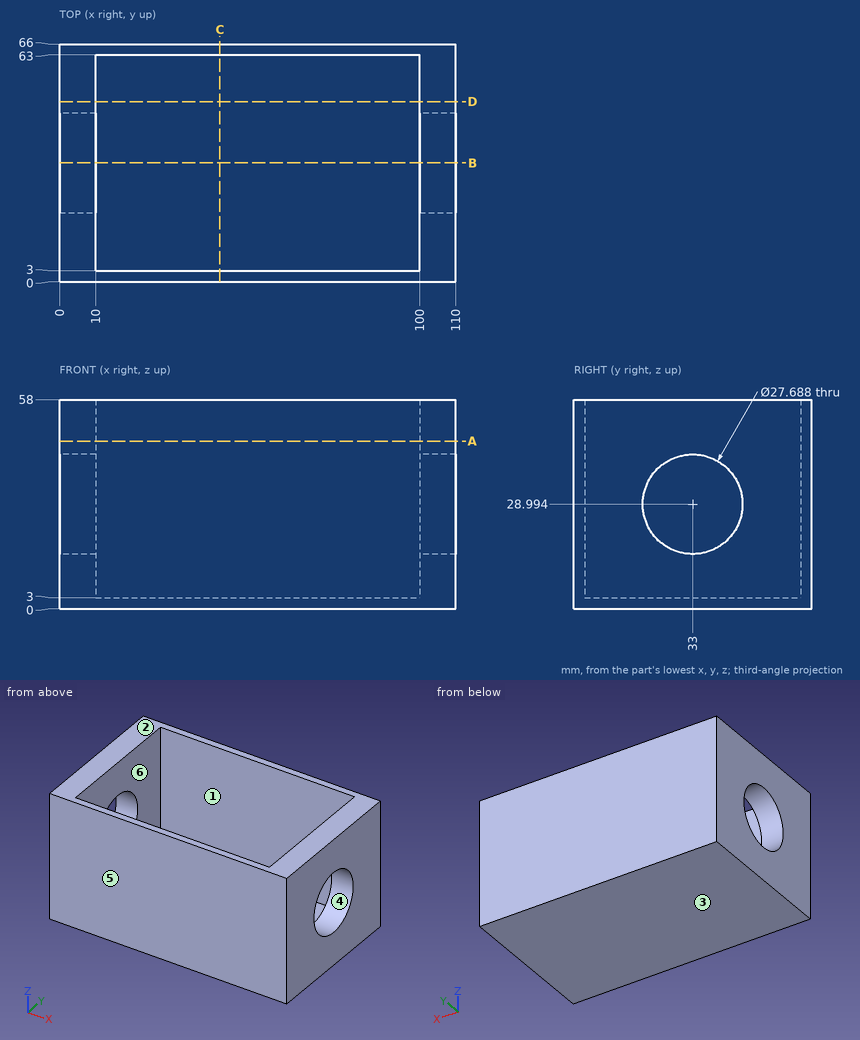
Here's the drawing with two shaded views (mm, measured from the low corner). I have some questions. A direction names the side the tool comes from. Round coordinates to 2 decimals unless told otherwise and drop trailing zeros. Loops run counter-clockwise (first coordinate to the right, second up) from the corner with the lowest first, then second, coordinate; pieces in that order, holes last. Notation, with made-up numbers: (-15, 34) - (37, 34) arc R25 cw to (37, 55) - close; hole circle Ø3 at (21, 1.25). An arc over 180 degrees is marked (long way). Write item = value, one per line.
1) Imagine slicing it at B-B (y = 33). Please give me the cut outline in (x, z).
Computed:
outline = (0, 0) - (110, 0) - (110, 15.15) - (100, 15.15) - (100, 3) - (10, 3) - (10, 15.15) - (0, 15.15) - close; (0, 42.84) - (10, 42.84) - (10, 58) - (0, 58) - close; (100, 42.84) - (110, 42.84) - (110, 58) - (100, 58) - close
2) Imagine slicing it at C-C (x = 44.5). Please give me the cut outline in (y, z).
Computed:
outline = (0, 0) - (66, 0) - (66, 58) - (63, 58) - (63, 3) - (3, 3) - (3, 58) - (0, 58) - close
3) Imagine slicing it at A-A (z = 46.5). Please give me the cut outline in (x, y), and give its area (3 significant figures).
Computed:
outline = (0, 0) - (110, 0) - (110, 66) - (0, 66) - close; hole (10, 3) - (100, 3) - (100, 63) - (10, 63) - close
area = 1,860 mm2
4) I'm going to push flat-ended pins straight in: P1, Ø8, axis at x = 89, y = 54.5, coming from the +Z side; P2, Ø16.5, axis at y = 44, z = 18, coming from the -X side. Where does each tip first touch, or does it pass through?
Computed:
P1 = 3
P2 = 0
5) Imagine slicing it at D-D (y = 50). Please give me the cut outline in (x, z).
Computed:
outline = (0, 0) - (110, 0) - (110, 58) - (100, 58) - (100, 3) - (10, 3) - (10, 58) - (0, 58) - close
6) If we mould it in two halves opening along Z, with no side actions, what happens to the marked faces 1, 2, 3 and 4? For each: pulls with the +Z half, pulls with the -Z half, needs draft (parallel to the pull), parting line crosses it, or undercut.
Computed:
face_1 = needs draft
face_2 = pulls with the +Z half
face_3 = pulls with the -Z half
face_4 = undercut
7) On a 3-axis mill with a long thin cutter (end or side, diameter ignored), from which of +Z, -Z, +X, -X, +Y, -Y can I reach the whole of each face in a straight line? I mean the marked faces 5 and 6. Say none if no direction works.
Computed:
face_5 = +Z, -Z, +X, -X, -Y
face_6 = +Z
8) I need wall thicknesses on line 1 along X through (y, z) = (40.5, 10.5); line 2 along Y through (x, z) = (73, 41.5); line 3 along Z through (x, y) = (106.75, 33). Which ranges of each line are inside material? Lowest first, please. Write a range as from..to.
Computed:
line_1 = 0..10, 100..110
line_2 = 0..3, 63..66
line_3 = 0..15.15, 42.84..58
